from build123d import *

# Parameters (mm, degrees)
EXTRUDE_1_DEPTH     = 100
SKETCH_2_R          = 1.5
CUT_EXTRUDE_1_DEPTH = 10
CUT_EXTRUDE_START   = -10
SKETCH_3_R          = 1.5
CUT_EXTRUDE_2_DEPTH = 10


with BuildPart() as part:
    # Эскиз1 → Бобышка-Вытянуть1 (new body)
    with BuildSketch(Plane.XY):
        Polygon((1.58771324, -2.75), (3.175426481, 0), (1.58771324, 2.75), (-1.58771324, 2.75), (-3.175426481, 0), (-1.58771324, -2.75), align=None)
    extrude(amount=EXTRUDE_1_DEPTH)

    # Эскиз2 → Вырез-Вытянуть1 (cut)
    with BuildSketch(Plane(origin=(0, 0, 0), x_dir=(-1, 0, 0), z_dir=(0, 0, -1))):
        Circle(SKETCH_2_R)
    extrude(amount=-CUT_EXTRUDE_1_DEPTH, mode=Mode.SUBTRACT)

    # Эскиз3 → Вырез-Вытянуть2 (cut)
    with BuildSketch(Plane.XY.offset(100).offset(CUT_EXTRUDE_START)):
        with Locations(Location((0, 0, 0), (0, 0, 180))):
            Circle(SKETCH_3_R)
    extrude(amount=CUT_EXTRUDE_2_DEPTH, mode=Mode.SUBTRACT)


solid = part.part
Model file for the job. Use its own axes, mm. A direction names the side the tool comes from. Coordinates: 2 decimals unless noted, no trailing zeros. Order: outer loops, then holes, each group sorted by start corner. A loop starts at its lowest first (then second) coordinate and runs counter-clockwise, first axis right, second up. Notation, with made-up numbers: M 86,-4.75 L 90,-4.75 A34 ccw 90,26.25 Z; hole C 17.5,19.25 d9. An arc over 180 degrees is marked long. Return JSON: item names as keys, results as strings.
1. Drill centre lines: probe 1 along Y at (x, z) = (0, 6.75); probe 2 along Z at (x, y) = (0.5, 0.3); probe 3 along Y at (x, z) = (0.5, 95.5). Where is each one in solid material? Low to high.
Ans:
{"probe 1": "-2.75 to -1.5, 1.5 to 2.75", "probe 2": "10 to 90", "probe 3": "-2.75 to -1.41, 1.41 to 2.75"}
2. Saw through at A-A (z = 7). Give the cut face in (x, y).
Ans:
{"outline": "M -3.18,0 L -1.59,-2.75 L 1.59,-2.75 L 3.18,0 L 1.59,2.75 L -1.59,2.75 Z; hole C 0,0 d3"}
3. Flat gauge pins, fed straight in: pin 1 (0.9 mm diameter, centred on x = 0, y = 0, fed in from -Z); pin 2 (3 mm diameter, centred on x = -2.5, y = -1.5, fed in from +Z); pin 3 (1 mm diameter, centred on y = -2, z = 43.5, fed in from -X). Where does each tip first touch, or does it go through?
Ans:
{"pin 1": "z = 10", "pin 2": "z = 100", "pin 3": "x = -2.31"}
4. Pull direction Y, two halves, no side cores. Call faces 4 (the face through (1.4, 1.3, 100)), 5 (the face through (-2.37, 1.394, 49.3)), 6 (the face through (0, 0, 10)): +Y half, -Y half, draft (parallel to the pull), parting line (faces both ways), or undercut.
Ans:
{"face 4": "draft", "face 5": "+Y half", "face 6": "undercut"}
5. Saw through at B-B (x = 0). Give the cut face in (y, z).
Ans:
{"outline": "M -2.75,0 L -1.5,0 L -1.5,10 L 1.5,10 L 1.5,0 L 2.75,0 L 2.75,100 L 1.5,100 L 1.5,90 L -1.5,90 L -1.5,100 L -2.75,100 Z"}
6. Tool access for faces 1 (the face through (1.5, 0.07, 4.93)), 2 (the face through (2.37, -1.394, 49.3)), 3 (the face through (0, 0, 90)): list every direction of +Z, -Z, +X, -X, +Y, -Y with a clear straight run to the whole face (end or side of a thin tool).
Ans:
{"face 1": "-Z", "face 2": "+Z, -Z, +X, -Y", "face 3": "+Z"}
7. Saw through at C-C (z = 76.5). Give the cut face in (x, y), and give its area (3 significant figures).
Ans:
{"outline": "M -3.18,0 L -1.59,-2.75 L 1.59,-2.75 L 3.18,0 L 1.59,2.75 L -1.59,2.75 Z", "area": "26.2 mm^2"}
